Input: part model. Units: mm. Frame: model coordinates. Coordinates: 2 decimals unless noted, no trailing zeros. Loops run counter-clockwise (first coordinate to the right, second up) from the corner with the lowest first, then second, coordinate; pieces in that order, holes last.
```python
from build123d import *

# Parameters (mm, degrees)
SKETCH1_R           = 0.25
BOSS_EXTRUDE1_DEPTH = 0.6
SKETCH2_R           = 0.25
CUT_EXTRUDE1_DEPTH  = 1.6


with BuildPart() as part:
    # Sketch1 → Boss-Extrude1 (new body)
    with BuildSketch(Plane(origin=(0, 0, 0), x_dir=(1, 0, 0), z_dir=(0, 1, 0))):
        with BuildLine():
            Line((2.454545455, 3.424242424), (2.454545455, 10.818181818))
            ThreePointArc((2.454545455, 10.818181818), (1.848484848, 11.424242424), (1.242424242, 10.818181818))
            Line((1.242424242, 10.818181818), (1.242424242, 3.424242424))
            Line((1.242424242, 3.424242424), (-4.151515152, 3.424242424))
            ThreePointArc((-4.151515152, 3.424242424), (-4.506914305, 3.309100243), (-4.727272727, 3.007424182))
            Line((-4.727272727, 3.007424182), (-4.727272727, 2.628939455))
            ThreePointArc((-4.727272727, 2.628939455), (-4.506914305, 2.327263393), (-4.151515152, 2.212121212))
            Line((-4.151515152, 2.212121212), (1.242424242, 2.212121212))
            Line((1.242424242, 2.212121212), (1.242424242, -5.181818182))
            ThreePointArc((1.242424242, -5.181818182), (1.848484848, -5.787878788), (2.454545455, -5.181818182))
            Line((2.454545455, -5.181818182), (2.454545455, 2.212121212))
            Line((2.454545455, 2.212121212), (7.848484848, 2.212121212))
            ThreePointArc((7.848484848, 2.212121212), (8.454545455, 2.818181818), (7.848484848, 3.424242424))
            Line((7.848484848, 3.424242424), (2.454545455, 3.424242424))
        make_face()
        with Locations((1.848484848, 10.818181818)):
            Circle(SKETCH1_R, mode=Mode.SUBTRACT)
        with Locations((1.848484848, -5.181818182)):
            Circle(SKETCH1_R, mode=Mode.SUBTRACT)
        with Locations((-4.151515152, 2.818181818)):
            Circle(SKETCH1_R, mode=Mode.SUBTRACT)
        with Locations((7.848484848, 2.818181818)):
            Circle(SKETCH1_R, mode=Mode.SUBTRACT)
    extrude(amount=BOSS_EXTRUDE1_DEPTH)

    # Sketch2 → Cut-Extrude1 (cut, through all)
    with BuildSketch(Plane(origin=(0, 0.6, 0), x_dir=(1, 0, 0), z_dir=(0, 1, 0))):
        with Locations((1.848484848, 2.818181818)):
            Circle(SKETCH2_R)
    extrude(amount=-CUT_EXTRUDE1_DEPTH, mode=Mode.SUBTRACT)


solid = part.part
```
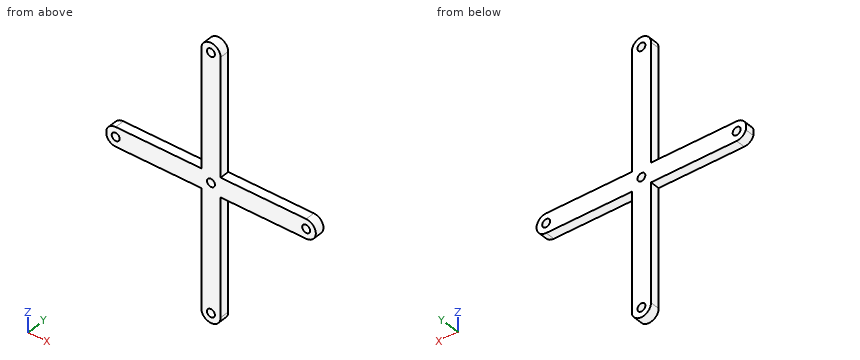
Item 1: Contact query for a flat-ended pin moving along its axis: P1, Ø1.5, axis at x = 4, z = -6, coming from the +Y side. Output: stop coordinate, or through.
Result:
P1: passes through
Item 2: Section query C-C (x = 7). Output: boundary loops of the cut face in (y, z).
Result:
outline: (0, -3.42) - (0.6, -3.42) - (0.6, -2.21) - (0, -2.21) - close
Item 3: Line query: L1, parallel to X at y = 0.15, z = 4; L2, parallel to Z at x = 3, y = 0.35. Output: solid intervals per line, ascending.
Result:
L1: x = 1.24 to 2.45
L2: z = -3.42 to -2.21
Item 4: Section query B-B (z = 4.5). Output: boundary loops of the cut face in (x, y), then the cut area to 3 significant figures.
Result:
outline: (1.24, 0) - (2.45, 0) - (2.45, 0.6) - (1.24, 0.6) - close
area: 0.727 mm2
Item 5: Section query A-A (y = 0.35). Output: boundary loops of the cut face in (x, z), then the cut area to 3 significant figures.
Result:
outline: (-4.73, -3.01) arc R0.61 ccw to (-4.15, -3.42) - (1.24, -3.42) - (1.24, -10.82) arc R0.61 ccw to (2.45, -10.82) - (2.45, -3.42) - (7.85, -3.42) arc R0.61 ccw to (7.85, -2.21) - (2.45, -2.21) - (2.45, 5.18) arc R0.61 ccw to (1.24, 5.18) - (1.24, -2.21) - (-4.15, -2.21) arc R0.61 ccw to (-4.73, -2.63) - close; hole circle Ø0.5 at (-4.15, -2.82); hole circle Ø0.5 at (1.85, -10.82); hole circle Ø0.5 at (1.85, -2.82); hole circle Ø0.5 at (1.85, 5.18); hole circle Ø0.5 at (7.85, -2.82)
area: 33.8 mm2
